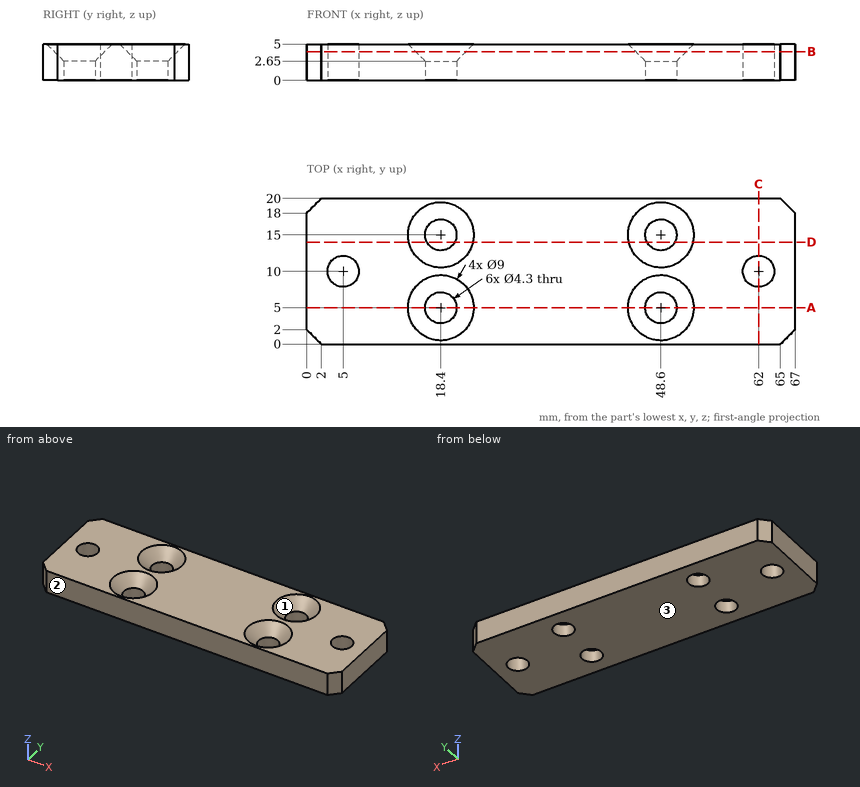
The figure shows three views and two pictorial views of one solid part (mm, origin at its lowest corner). Answer the questions. Give positions to 0.01 mm unless a question says otherwise; leave off trailing zeros. Order: outer loops, then holes, each group sorted by start corner. A loop starts at its lowest first (then second) coordinate and runs counter-clockwise, first axis right, second up. Notation, with made-up numbers: M 48,33 L 100,33 A23 ccw 100,43 Z; hole C 67,-33.5 d6. An arc over 180 degrees is marked long. Return JSON: item names as keys, results as strings.
Q1. The mould has two halves that part along Y. Classify the marked faces 1, 2 and 3: pulls with the +Y half, pulls with the -Y half, needs draft (parallel to the pull), parting line crosses it, or undercut.
Answer below:
{"face 1": "undercut", "face 2": "pulls with the -Y half", "face 3": "needs draft"}
Q2. Find section B-B, the plane z = 3.95. Write down the section's boundary in (x, y), and give its area (3 significant figures).
Answer below:
{"outline": "M 0,2 L 2,0 L 65,0 L 67,2 L 67,18 L 65,20 L 2,20 L 0,18 Z; hole C 5,10 d4.3; hole C 18.4,5 d6.9; hole C 18.4,15 d6.9; hole C 48.6,5 d6.9; hole C 48.6,15 d6.9; hole C 62,10 d4.3", "area": "1,150 mm^2"}
Q3. Find section A-A, the plane y = 5. Write down the section's boundary in (x, z), and give its area (3 significant figures).
Answer below:
{"outline": "M 0,0 L 16.25,0 L 16.25,2.65 L 13.9,5 L 0,5 Z; M 20.55,0 L 46.45,0 L 46.45,2.65 L 44.1,5 L 22.9,5 L 20.55,2.65 Z; M 50.75,0 L 67,0 L 67,5 L 53.1,5 L 50.75,2.65 Z", "area": "281 mm^2"}
Q4. Each of these flat-tipped pins is pushed along its axis until it touches: pin 1 (4 mm diameter, centred on x = 18.4, y = 15, fed in from -Z); pin 2 (5 mm diameter, centred on x = 48.6, y = 5, fed in from +Z). Where does it stop, or does it pass through?
Answer below:
{"pin 1": "passes through", "pin 2": "stops at z = 3"}
Q5. Find section D-D, the plane y = 14. State how many separate pieces and enclosed holes the cut face has, and give its area (3 significant figures).
Answer below:
{"separate pieces": "3", "enclosed holes": "0", "area": "285 mm^2"}
Q6. Find section C-C, the plane x = 62. Write down the section's boundary in (y, z), and give its area (3 significant figures).
Answer below:
{"outline": "M 0,0 L 7.85,0 L 7.85,5 L 0,5 Z; M 12.15,0 L 20,0 L 20,5 L 12.15,5 Z", "area": "78.5 mm^2"}
Q7. Find the intervals of material crossed by line 1 along Y through (x, z) = (18.4, 1.9); line 2 along X through (y, z) = (15, 0.95); line 3 along X through (y, z) = (14.25, 2.15), in increasing order. Write a range as [from, to].
Answer below:
{"line 1": "y = [0, 2.85], [7.15, 12.85], [17.15, 20]", "line 2": "x = [0, 16.25], [20.55, 46.45], [50.75, 67]", "line 3": "x = [0, 16.39], [20.41, 46.59], [50.61, 67]"}
